Part model, mm, in its own coordinate system. Round coordinates to 2 decimals unless told otherwise and drop trailing zeros. Write each loop counter-clockwise with the first axis right and the second up, starting at its lowest first coordinate (ties: lowest second). Pieces come first, ordered by that corner, then holes. Notation, with made-up numbers: M 43.5,74.5 L 87.5,74.5 A22 cw 87.5,107.5 Z; hole C 6,62.25 d3. An arc over 180 degrees is marked long. Answer as a JSON object with one key per item and string values. Group by question number.
1. Band-saw the part on A-A, the plane x = 20. Write the cut outline in (y, z).
2. Drill centre lines: line 1 (Z direction, x = 23, y = 0.15); line 2 (X direction, y = -0.55, z = 1.4); line 3 (Y direction, x = 6, z = -1.5). Where is each one in solid material? Low to high. Write a range as from..to.
3. Drop flat-ended pins along their axis: pin 1 (1.5 mm diameter, centred on x = 23.5, z = -1.5, fed in from +Y); pin 2 (1 mm diameter, centred on x = 16.5, y = -1, fed in from +Z). Give the stop position or say it passes through.
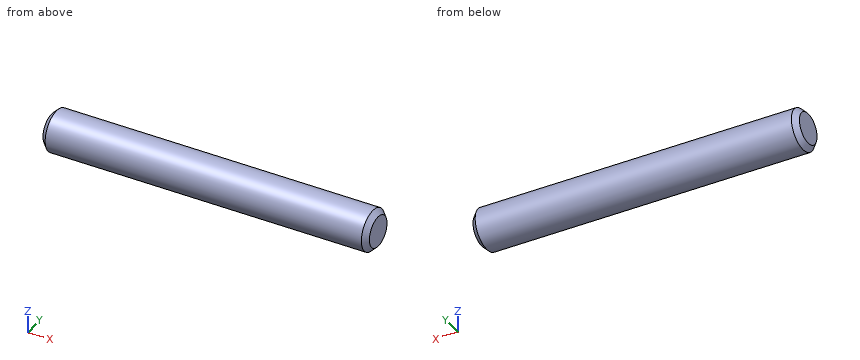
Autodesk Inventor part; units mm, degrees
ref_plane "Startebene" through (0, 0, 0) normal (1, 0, 0) x (0, 1, 0)
ref_plane "XZ Plane" through (0, 0, 0) normal (0, 1, 0) x (-1, 0, 0)
ref_plane "XY Plane" through (0, 0, 0) normal (0, 0, 1) x (1, 0, 0)
sketch "Hauptskizze" plane through (0, 0, 0) normal (0, 0, 1) x (1, 0, 0)
  line L0 (0, 0) -> (32, 0)
  line L1 (0, 0) -> (0, 2)
  line L2 (0, 2) -> (16, 2)
  line L3 (32, 2) -> (32, 0)
  line L4 (16, 2) -> (32, 2)
  dimension "d3" = 4
  dimension "d5" = 4
revolve "Umdrehung1" add sketch "Hauptskizze" angle 360 about axis through (0, 0, 0) along (1, 0, 0)
chamfer "Fase3" distance 0.5 angle 45 1 edges at (0, -2, 0) measured on face at (10.6667, 1.9741, -0.3208)
chamfer "Fase2" distance 0.5 angle 45 1 edges at (32, -2, 0) measured on face at (26.6667, 1.9935, -0.1609)
properties part number "Welle" material "Steel"
Worked answers:
{
 "1": {"outline": "C 0,0 d4"},
 "2": {"line 1": "z = -1.99..1.99", "line 2": "x = 0..32", "line 3": "y = -1.32..1.32"},
 "3": {"pin 1": "stops at y = 1.85", "pin 2": "stops at z = 1.94"}
}
